Read the model definition and answer for the solid it produces. Units are mm, in the model's axes. A direction names the side the tool comes from. Coordinates: 2 decimals unless noted, no trailing zeros. Order: outer loops, then holes, each group sorted by start corner. A loop starts at its lowest first (then second) coordinate and runs counter-clockwise, first axis right, second up. Notation, with made-up numbers: (11.25, 74) -> (44.25, 74) arc R21 ccw to (44.25, 86) -> close; hole circle Ø8 at (20.5, 28.5). An arc over 180 degrees is marked (long way). Answer in a Markdown table with one row per item.
from build123d import *

# Parameters (mm, degrees)
BOSS_EXTRUDE1_DEPTH = 177.8
CUT_EXTRUDE1_DEPTH  = 50.8


with BuildPart() as part:
    # Sketch1 → Boss-Extrude1 (new body)
    with BuildSketch(Plane(origin=(0, 0, 0), x_dir=(1, 0, 0), z_dir=(0, 1, 0))):
        Polygon((308.61, 400.05), (203.2, 400.05), (203.2, 146.05), (-203.2, 146.05), (-203.2, 400.05), (-308.61, 400.05), (-308.61, -400.05), (308.61, -400.05), align=None)
    extrude(amount=BOSS_EXTRUDE1_DEPTH)

    # Sketch2 → Cut-Extrude1 (cut)
    with BuildSketch(Plane.XZ):
        Polygon((308.61, -400.05), (275.513805506, -400.05), (275.513805506, 367.013597839), (-275.682759314, 367.013597839), (-275.682759314, -400.05), (-308.61, -400.05), (-308.61, 400.05), (-275.682759314, 400.05), (275.513805506, 400.05), (308.61, 400.05), align=None)
    extrude(amount=-CUT_EXTRUDE1_DEPTH, mode=Mode.SUBTRACT)


solid = part.part
Q1. The part is cut by section B-B (y = 64.5). Write down the section's boundary in (x, z).
Outcome:
| item | result |
|---|---|
| outline | (-308.61, -400.05) -> (-203.2, -400.05) -> (-203.2, -146.05) -> (203.2, -146.05) -> (203.2, -400.05) -> (308.61, -400.05) -> (308.61, 400.05) -> (-308.61, 400.05) -> close |
Q2. The part is cut by section C-C (x = 102.5). Write down the section's boundary in (y, z), then the cut area to 3 significant figures.
Outcome:
| item | result |
|---|---|
| outline | (0, -146.05) -> (177.8, -146.05) -> (177.8, 400.05) -> (50.8, 400.05) -> (50.8, 367.01) -> (0, 367.01) -> close |
| area | 95,400 mm² |
Q3. The part is cut by section A-A (z = -246.5). Write down the section's boundary in (x, y), then the cut area to 3 significant figures.
Outcome:
| item | result |
|---|---|
| outline | (-308.61, 50.8) -> (-275.68, 50.8) -> (-275.68, 0) -> (-203.2, 0) -> (-203.2, 177.8) -> (-308.61, 177.8) -> close; (203.2, 0) -> (275.51, 0) -> (275.51, 50.8) -> (308.61, 50.8) -> (308.61, 177.8) -> (203.2, 177.8) -> close |
| area | 34,100 mm² |
Q4. For a pull along X with two mould halves and no side action, classify faces 1 (the face through (-203.2, 88, -271)), 2 (the face through (276, 50.8, 91)), 3 (the face through (-308.61, 113, -6)) as pulls with the +X half, pulls with the -X half, needs draft (parallel to the pull), parting line crosses it, or undercut.
Outcome:
| item | result |
|---|---|
| face 1 | undercut |
| face 2 | needs draft |
| face 3 | pulls with the -X half |
Q5. For faces 4 (the face through (3, 88, -146.05)), 5 (the face through (275.514, 25, -22)), 6 (the face through (-275.683, 25, -11)), 7 (the face through (4, 25, 367.014)), 8 (the face through (-255, 88, -400.05)), determine the directions among +Z, -Z, +X, -X, +Y, -Y from which every point of the face is accessible in a straight line to the end or side of a thin tool.
Outcome:
| item | result |
|---|---|
| face 4 | -Z, +Y, -Y |
| face 5 | +Z, -Z, +X, -Y |
| face 6 | +Z, -Z, -X, -Y |
| face 7 | +Z, +X, -X, -Y |
| face 8 | -Z, +X, -X, +Y, -Y |
Q6. Consider line 1 (X direction, y = 161, z = -347); line 2 (Z direction, x = -35, y = 35.5); line 3 (Z direction, x = -113, y = 170). Determine where each line is inside the solid, lowest interval first.
Outcome:
| item | result |
|---|---|
| line 1 | -308.61 to -203.2, 203.2 to 308.61 |
| line 2 | -146.05 to 367.01 |
| line 3 | -146.05 to 400.05 |
Q7. Given pin 1 (12 mm diameter, centred on x = -135.5, y = 32.5, fed in from -Z), flat-ended and moving along its own axis, determine where the tip first touches the part or whether it passes through.
Outcome:
| item | result |
|---|---|
| pin 1 | z = -146.05 |
Q8. The part is cut by section D-D (z = 109). Write down the section's boundary in (x, y).
Outcome:
| item | result |
|---|---|
| outline | (-308.61, 50.8) -> (-275.68, 50.8) -> (-275.68, 0) -> (275.51, 0) -> (275.51, 50.8) -> (308.61, 50.8) -> (308.61, 177.8) -> (-308.61, 177.8) -> close |
